Drawing for the job (mm, zero at the part's lowest x, y, z). A direction names the side the tool comes from. Round coordinates to 2 decimals unless told otherwise and drop trailing zeros. Write each loop counter-clockwise with the first axis right and the second up, starting at its lowest first coordinate (ties: lowest second). Pieces come first, ordered by that corner, then holes. Notation, with made-up numbers: (32.5, 35.5) - (81.5, 35.5) arc R16 ccw to (81.5, 53.5) - close; hole circle Ø5 at (-4, 82.5). An arc over 180 degrees is marked (long way). Answer in a Markdown table with one row per item.
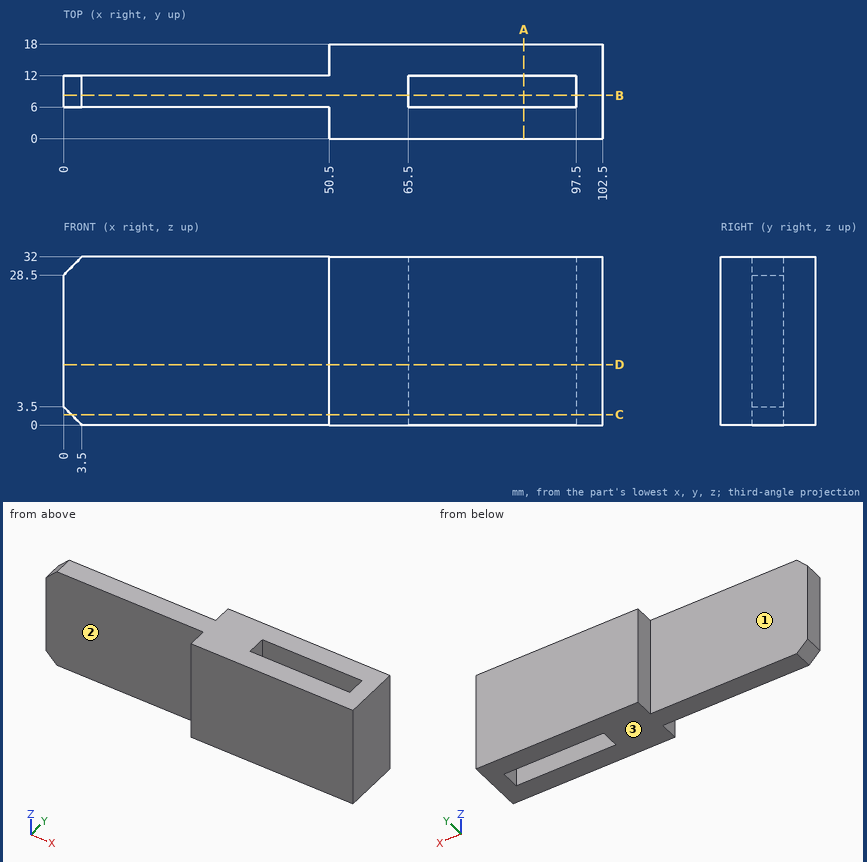
Q1. Saw through at D-D on z = 11.5. List the corners of the cut face in (x, y).
Computed:
| item | result |
|---|---|
| outline | (0, 6) - (50.5, 6) - (50.5, 0) - (102.5, 0) - (102.5, 18) - (50.5, 18) - (50.5, 12) - (0, 12) - close; hole (65.5, 6) - (97.5, 6) - (97.5, 12) - (65.5, 12) - close |
Q2. Flat gauge pins, fed straight in: pin 1 (5 mm diameter, centred on x = 15.5, z = 17, fed in from -Y); pin 2 (3 mm diameter, centred on y = 16, z = 9.5, fed in from -X); pin 3 (5 mm diameter, centred on x = 33.5, y = 2, fed in from -Z) (3 decimals); pin 4 (16 mm diameter, centred on x = 14, z = 14.5, fed in from +Y). Where does each tip first touch, or does it go through?
Computed:
| item | result |
|---|---|
| pin 1 | stops at y = 6 |
| pin 2 | stops at x = 50.5 |
| pin 3 | passes through |
| pin 4 | stops at y = 12 |
Q3. Drill centre lines: line 1 (Y direction, x = 84, z = 14); line 2 (X direction, y = 7.75, z = 28); line 3 (X direction, y = 1, z = 5.5). Where is each one in solid material? Low to high.
Computed:
| item | result |
|---|---|
| line 1 | y = 0 to 6, 12 to 18 |
| line 2 | x = 0 to 65.5, 97.5 to 102.5 |
| line 3 | x = 50.5 to 102.5 |
Q4. Saw through at B-B on y = 8.25. List the corners of the cut face in (x, z).
Computed:
| item | result |
|---|---|
| outline | (0, 3.5) - (3.5, 0) - (65.5, 0) - (65.5, 32) - (3.5, 32) - (0, 28.5) - close; (97.5, 0) - (102.5, 0) - (102.5, 32) - (97.5, 32) - close |
Q5. 3-axis set-ups, long thin cutter, end or side, ignore diameter. For the marked faces 1, 2 and 3: which of +Z, -Z, +X, -X, +Y, -Y reach the whole face in a straight line?
Computed:
| item | result |
|---|---|
| face 1 | +Z, -Z, -X, +Y |
| face 2 | +Z, -Z, -X, -Y |
| face 3 | -Z, +X, -X, +Y, -Y |
Q6. Saw through at A-A on x = 87.5. List the corners of the cut face in (y, z), then the cut area to 3 significant figures.
Computed:
| item | result |
|---|---|
| outline | (0, 0) - (6, 0) - (6, 32) - (0, 32) - close; (12, 0) - (18, 0) - (18, 32) - (12, 32) - close |
| area | 384 mm2 |
Q7. Saw through at C-C on z = 2. List the corners of the cut face in (x, y), then the cut area to 3 significant figures.
Computed:
| item | result |
|---|---|
| outline | (1.5, 6) - (50.5, 6) - (50.5, 0) - (102.5, 0) - (102.5, 18) - (50.5, 18) - (50.5, 12) - (1.5, 12) - close; hole (65.5, 6) - (97.5, 6) - (97.5, 12) - (65.5, 12) - close |
| area | 1,040 mm2 |
